Input: part model. Units: mm. Frame: model coordinates. A direction names the side the tool comes from. Round coordinates to 2 decimals unless told otherwise and drop trailing zeros. Write each loop counter-clockwise with the first axis right and the second up, starting at its lowest first coordinate (ties: lowest second). Pieces come first, ordered by that corner, then holes. Notation, with made-up numbers: (4.5, -8.5) -> (46.5, -8.5) arc R12 ccw to (46.5, 10.5) -> close; hole circle Ø5 at (51.25, 54.25). An arc over 180 degrees is marked (long way). Write item = value, one per line.
```python
from build123d import *

# Parameters (mm, degrees)
F0_R           = 2
F1_DEPTH       = 20
F3_W           = 10.25
F3_H           = 12
F4_DEPTH       = 10.501
F5_R           = 2
F7_D           = 5
F7_CSINK_D     = 11
F7_CSINK_ANGLE = 90


# Not quite as in the source:
# - a pattern or mirror of a feature is missing from the dataset's text; its kind, count and spacing are read off the source's solid


with BuildPart() as f1:
    # F0 (on Right) → F1 (new body, symmetric)
    with BuildSketch(Plane.YZ):
        with BuildLine():
            Line((0, 5), (0, 0))
            Line((0, 0), (30, 0))
            Line((30, 0), (30, 10))
            ThreePointArc((30, 10), (33.5355339059, 18.5355339059), (25, 15))
            Line((25, 15), (25, 5))
            Line((25, 5), (0, 5))
        make_face()
        with Locations((30, 15)):
            Circle(F0_R, mode=Mode.SUBTRACT)
    extrude(amount=F1_DEPTH, both=True)

    # F3 (on offset) → F4 (cut, through all)
    with BuildSketch(Plane.XY.offset(9.5)):
        with Locations((14.875, 31)):
            Rectangle(F3_W, F3_H)
    f4 = extrude(amount=F4_DEPTH, mode=Mode.SUBTRACT)

    # F4_copies: F4 across plane
    add(f4.mirror(Plane(origin=(0, 0, 0), x_dir=(0, 0, -1), z_dir=(-1, 0, 0))), mode=Mode.SUBTRACT)

    # F5
    f5_edges = [f1.edges().sort_by_distance(p)[0] for p in [
        (0, 25, 5),
    ]]
    fillet(f5_edges, radius=F5_R)

    # F7 (through all)
    with Locations(Plane(origin=(0, 0, 0), x_dir=(1, 0, 0), z_dir=(0, 0, -1))):
        with Locations((-12.5, -10), (0, -15), (12.5, -10)):
            CounterSinkHole(F7_D / 2, F7_CSINK_D / 2, counter_sink_angle=F7_CSINK_ANGLE)


solid = f1.part
```
1) Access query for faces 1 (the face through (-15, 28, 9.5)), 2 (the face through (0, 12, 5)), 3 (the face through (15, 28, 9.5)). Directions: +Z, -Z, +X, -X, +Y, -Y. A direction counts if a zero-diameter tool reaches every point of the face in a straight line with its end or side. Return the directions, or none.
Solutions:
face_1 = +Z, -X, +Y, -Y
face_2 = +Z, +X, -X, -Y
face_3 = +Z, +X, +Y, -Y
2) First-contact query: P1, Ø5, axis at y = 30, z = 15, coming from the +X side; P2, Ø8, axis at x = 8.5, z = 3.5, coming from the +Y side; P3, Ø11.5, axis at x = 5.5, y = 14, coming from the +Z side. Flat tips, straight axial feed; report the tip coordinate or a pass-through.
Solutions:
P1 = 9.75
P2 = 30
P3 = 5
3) Line query: L1, parallel to Y at x = -1.25, z = 15; L2, parallel to Y at x = 0, z = 4.1; L3, parallel to X at y = 15, z = 4.25. Output: solid intervals per line, ascending. Write a range as from..to.
Solutions:
L1 = 25..28, 32..35
L2 = 0..12.5, 17.5..30
L3 = -20..-2.5, 2.5..20
4) Draft query along X for faces 4 (the face through (-0.136, 31.908, 15.601)), 5 (the face through (0.54, 17.44, 4.01)), 6 (the face through (20, 15, 3)). Return one class per face: +X half, -X half, draft (parallel to the pull), parting line (faces both ways), or undercut.
Solutions:
face_4 = draft
face_5 = undercut
face_6 = +X half
5) Cut plane A-A (x = 0). Return the cut outline in (y, z).
Solutions:
outline = (0, 0) -> (9.5, 0) -> (12.5, 3) -> (12.5, 5) -> (0, 5) -> close; (17.5, 3) -> (20.5, 0) -> (30, 0) -> (30, 10) arc R5 ccw (long way) to (25, 15) -> (25, 7) arc R2 cw to (23, 5) -> (17.5, 5) -> close; hole circle Ø4 at (30, 15)
6) Cut plane B-B (z = 2). Return the cut outline in (x, y), and give its area (3 significant figures).
Solutions:
outline = (-20, 0) -> (20, 0) -> (20, 30) -> (-20, 30) -> close; hole circle Ø7 at (-12.5, 10); hole circle Ø7 at (0, 15); hole circle Ø7 at (12.5, 10)
area = 1,080 mm^2
7) Cut plane D-D (y = 10). Count the separate pieces of the cut face and the enclosed holes in it, and give its area (3 significant figures).
Solutions:
separate_pieces = 3
enclosed_holes = 0
area = 130 mm^2
8) Cut plane C-C (x = -12.5). Return the cut outline in (y, z).
Solutions:
outline = (0, 0) -> (4.5, 0) -> (7.5, 3) -> (7.5, 5) -> (0, 5) -> close; (12.5, 3) -> (15.5, 0) -> (30, 0) -> (30, 9.5) -> (25, 9.5) -> (25, 7) arc R2 cw to (23, 5) -> (12.5, 5) -> close
